The listing builds one solid part. Answer for the finished solid, in the listing's coordinates (mm). Face numbers are marked on the shaded views. Give positions to 0.01 mm unless a question says otherwise; leave off trailing zeros. Write each loop counter-clockwise with the first axis right and the second up, starting at its lowest first coordinate (ties: lowest second). Pieces come first, ordered by that corner, then holes. Notation, with made-up numbers: M 77.5,81.25 L 92.5,81.25 A12 cw 92.5,99.25 Z; hole C -21,-6.75 d8. An arc over 180 degrees is marked long. Answer as a JSON object with one key per item and string values.
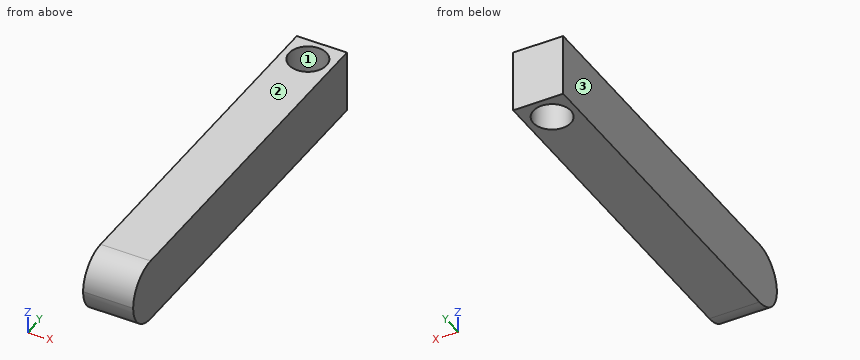
```python
from build123d import *

# Parameters (mm, degrees)
SKETCH1_W           = 80
SKETCH1_H           = 611.5
SKETCH1_R           = 30
BOSS_EXTRUDE1_DEPTH = 100
FILLET2_R           = 50


with BuildPart() as part:
    # Sketch1 → Boss-Extrude1 (new body)
    with BuildSketch(Plane.XY):
        with Locations((2.330379174, 234.720418357)):
            Rectangle(SKETCH1_W, SKETCH1_H)
        with Locations((2.330379174, 500.470418357)):
            Circle(SKETCH1_R, mode=Mode.SUBTRACT)
    extrude(amount=BOSS_EXTRUDE1_DEPTH)

    # Fillet2
    fillet2_edges = [part.edges().sort_by_distance(p)[0] for p in [
        (2.330379174, -71.029581643, 0),
        (2.330379174, -71.029581643, 100),
    ]]
    fillet(fillet2_edges, radius=FILLET2_R - 0.0001)  # a hair under: the kernel refuses the full size


solid = part.part
```
1. Flat-ended cylindrical pins translate along their axes: pin 1 (3 mm diameter, centred on x = -18.5, z = 59.5, fed in from -Y); pin 2 (5 mm diameter, centred on x = -26, z = 18.5, fed in from -Y); pin 3 (6 mm diameter, centred on x = 32.5, z = 64.5, fed in from -Y). Find the tip coordinate at first contact, or state that the pin passes through.
Verdict:
{"pin 1": "stops at y = -70.39", "pin 2": "stops at y = -61.76", "pin 3": "stops at y = -69.69"}
2. A cutting plane is placed at B-B, the plane z = 81. Give the vertices of the cut face in (x, y).
Verdict:
{"outline": "M -37.67,-60.26 L 42.33,-60.26 L 42.33,540.47 L -37.67,540.47 Z; hole C 2.33,500.47 d60"}
3. Consider line 1 along Y through (x, z) = (-20.5, 24); line 2 along Y through (x, z) = (-16.5, 67); line 3 along X through (y, z) = (496.5, 79.5). Determine where each line is inside the solid, lowest interval first.
Verdict:
{"line 1": "y = -63.74 to 481.01, 519.93 to 540.47", "line 2": "y = -68.05 to 477.12, 523.82 to 540.47", "line 3": "x = -37.67 to -27.41, 32.07 to 42.33"}
4. A cutting plane is placed at D-D, the plane z = 38.5. Give the vertices of the cut face in (x, y), plus the area to 3 significant figures.
Verdict:
{"outline": "M -37.67,-69.69 L 42.33,-69.69 L 42.33,540.47 L -37.67,540.47 Z; hole C 2.33,500.47 d60", "area": "46,000 mm2"}
5. The mould has two halves that part along X. Classify the marked faces 1, 2 and 3: released by +X, released by -X, zero draft, split by the parting line, or undercut.
Verdict:
{"face 1": "undercut", "face 2": "zero draft", "face 3": "released by -X"}
